Autodesk Inventor part; units mm, degrees
ref_plane "Plano de trabajo2" through (171, -60, 0) normal (1, 0, 0) x (0, 0, -1)
ref_plane "YZ Plane" through (0, 0, 0) normal (1, 0, 0) x (0, 1, 0)
ref_plane "XZ Plane" through (0, 0, 0) normal (0, 1, 0) x (-1, 0, 0)
sketch "Boceto7" plane through (0, 0, 0) normal (0, 0, 1) x (1, 0, 0)
  line L0 (0, 0) -> (342, 0)
  line L1 (171, 330.115) -> (171, 0) construction
  line L2 (131.5, 347.5309) -> (210.5, 347.5309) construction
  line L3 (210.5, 330.115) -> (131.5, 330.115)
  line L4 (0, 0) -> (131.5, 330.115)
  line L5 (342, 0) -> (210.5, 330.115)
  line L6 (0, 0) -> (0, -10) construction
  line L7 (0, -10) -> (78.602, -10) construction
  line L8 (0, -10) -> (78.602, -10)
  line L9 (0, -10) -> (0, 0)
  line L10 (78.602, -10) -> (342, -10)
  line L11 (342, -10) -> (342, 0)
  line L12 (131.5, 330.115) -> (131.5, 320.115)
  line L13 (131.5, 320.115) -> (210.5, 320.115)
  line L14 (210.5, 320.115) -> (210.5, 330.115)
  line L15 (78.602, -10) -> (78.602, 0)
  line L16 (263.398, -10) -> (263.398, 0)
  line L17 (0, -10) -> (78.602, -10)
  line L18 (78.602, -10) -> (78.602, -60)
  line L19 (78.602, -60) -> (0, -60)
  line L20 (0, -60) -> (0, -10)
  line L21 (263.398, -10) -> (263.398, -60)
  line L22 (263.398, -60) -> (342, -60)
  line L23 (342, -60) -> (342, -10)
  line L24 (78.602, 0) -> (116.5722, 189.115)
  line L25 (116.5722, 189.115) -> (225.4278, 189.115)
  line L26 (225.4278, 189.115) -> (263.398, 0)
  point P0 (263.398, 0)
  point P1 (263.398, -10)
  dimension "d68" = 79
  dimension "d69" = 39.5
  dimension "d70" = 342
  dimension "d71" = 330.115
  dimension "d72" = 10
  dimension "d73" = 78.602
  dimension "d74" = 10
  dimension "d111" = 50
  dimension "d144" = 141
extrude "Extrusión5" add sketch "Boceto7" along normal blind 35 contours L4 L12 L13 L14 L5 L0 L26 L25 L24 | L0 L15 L8 L9 | L3 L14 L13 L12 | L8 L18 L19 L20 | L0 L11 L10 L16 | L10 L23 L22 L21
extrude "Extrusión6" add sketch "Boceto7" along normal blind 191 contours L0 L15 L8 L9 | L3 L14 L13 L12 | L0 L11 L10 L16
ref_plane "Plano de trabajo2" through (171, -60, 0) normal (1, 0, 0) x (0, 0, -1)
sketch "Boceto12" plane through (171, -60, 0) normal (1, 0, 0) x (0, 0, -1)
  line L0 (-35, 380.115) -> (-191, 380.115)
  line L1 (-191, 380.115) -> (-35, 249.2155)
  line L2 (-35, 390.115) -> (-35, 60)
  line L3 (-173.0135, 380.115) -> (-35, 264.3079)
  line L4 (-173.0135, 395.115) -> (-35, 279.3079)
  line L5 (-173.0135, 410.115) -> (-35, 294.3079)
  line L6 (-173.0135, 425.115) -> (-35, 309.3079)
  line L7 (-173.0135, 440.115) -> (-35, 324.3079)
  line L8 (-173.0135, 455.115) -> (-35, 339.3079)
  line L9 (-173.0135, 470.115) -> (-35, 354.3079)
  line L10 (-173.0135, 485.115) -> (-35, 369.3079)
  line L11 (-173.0135, 500.115) -> (-35, 384.3079)
  line L12 (-173.0135, 515.115) -> (-35, 399.3079)
  line L13 (-173.0135, 530.115) -> (-35, 414.3079)
  line L14 (-35, 60) -> (-35, 390.115)
  line L15 (138.0135, 380.115) -> (138.0135, 210.115) construction
  point P0 (0, 60)
  point P1 (-10, 338.3304)
  point P2 (-23.0135, 325.115)
  point P3 (-12.1268, 325.115)
  point P4 (-30, 350.1124)
  point P5 (-30.0031, 385.115)
  point P6 (-47.8794, 380.115)
  point P7 (-65.7557, 380.115)
  point P8 (-83.632, 380.115)
  point P9 (-101.5083, 380.115)
  point P10 (-119.3846, 380.115)
  point P11 (-137.2609, 380.115)
  point P12 (-155.1372, 380.115)
  dimension "d90" = 40
  dimension "d93" = 15
  dimension "d107" = 170
  dimension "d108" = 0
extrude "Extrusión9" add sketch "Boceto12" along normal mid plane 79 contours L3 L2 L1 L0 | L0 L5 L2 L4 | L0 L7 L2 L6 | L0 L9 L2 L8 | L0 L2 L10
sketch "Boceto13" plane through (0, 0, 35) normal (0, 0, 1) x (1, 0, 0)
  circle A0 centre (81.5, 169.115) radius 12.7
  circle A1 centre (66.5, 119.115) radius 12.7
  circle A2 centre (51.5, 69.115) radius 12.7
  line L0 (116.5722, 189.115) -> (225.4278, 189.115)
  line L1 (131.5, 189.2155) -> (131.5, 320.115)
  line L2 (131.5, 320.115) -> (210.5, 320.115) construction
  line L3 (171, 320.115) -> (171, 34.3684) construction
  circle A3 centre (260.5, 169.115) radius 12.7
  circle A4 centre (275.5, 119.115) radius 12.7
  circle A5 centre (290.5, 69.115) radius 12.7
  point P0 (131.5, 193.411)
  dimension "d126" = 25.4
  dimension "d127" = 25.4
  dimension "d128" = 25.4
  dimension "d129" = 20
  dimension "d130" = 50
  dimension "d131" = 50
  dimension "d132" = 50
  dimension "d133" = 65
  dimension "d134" = 80
extrude "Extrusión10" cut sketch "Boceto13" against normal up to surface (35 mm away)
sketch "Boceto16" plane through (342, -60, 0) normal (1, 0, 0) x (0, 0, -1)
  line L0 (-191, 50) -> (-191, 60)
  line L1 (0, 0) -> (-35, 0)
  line L2 (-191, 50) -> (-35, 0)
  line L3 (-35, 0) -> (-35, 50)
  line L4 (-191, 62) -> (-35, 12)
  line L5 (-191, 74) -> (-35, 24)
  line L6 (-191, 86) -> (-35, 36)
  line L7 (-191, 98) -> (-35, 48)
  line L8 (-191, 110) -> (-35, 60)
  line L9 (-35, 50) -> (-191, 50)
  point P0 (0, 60)
  point P1 (-78.68, 50)
  point P2 (-116.12, 50)
  point P3 (-153.56, 50)
  dimension "d137" = 12
extrude "Extrusión13" add sketch "Boceto16" against normal blind 79 contours L9 L4 L3 L2 | L9 L6 L3 L5
mirror "Simetría2" about plane through (171, -60, 0) normal (1, 0, 0) of "Extrusión13"
thread "Rosca1"
thread "Rosca2"
thread "Rosca3"
thread "Rosca4"
thread "Rosca5"
thread "Rosca6"
properties part number "Soporte" material "Acero inoxidable 302 AISI"
For this review, take the finished solid that the model builds, in its own axes (mm). A direction names the side the tool comes from. Round coordinates to 2 decimals unless told otherwise and drop trailing zeros. Write each loop counter-clockwise with the first axis right and the second up, starting at its lowest first coordinate (ties: lowest second). Pieces come first, ordered by that corner, then holes. Notation, with made-up numbers: (43, 8) -> (95, 8) arc R25 ccw to (95, 43) -> close; hole circle Ø6 at (61.5, 74.5). An arc over 180 degrees is marked (long way). One line per question, with ' | ' between items. Start each with the question number.
1) Add section C-C (z = 26.5). Write out the cut boundary in (x, y) (3 decimals), and give its area (3 significant figures).
2) Wall thickness on line 1 along Y through (x, z) = (17, 48); line 2 along Y through (x, z) = (309, 59); line 3 along X through (y, z) = (-3, 13): over which ranges is each line inside the solid? List them lowest first.
3) Add section D-D (x = 241.5). Write out the cut boundary in (y, z), and give its area (3 significant figures).
4) Add section B-B (y = 32.5). Write out the cut boundary in (x, z), and give its area (3 significant figures).
5) Add section A-A (y = 161). Write out the cut boundary in (x, z), and give its area (3 significant figures).
6) Machinability: for faces 1 (the flat face through (263, -21, 67)), 2 (the flat face through (39, 0, 112)), 3 (the flat face through (78.602, -8, 53)), which of the approach directions +Z, -Z, +X, -X, +Y, -Y give a long, thin tool a straight path to every point of the face, cutting with its end or side? Answer none if there is none.
7) Mouldability with a two-part tool opening along Z and no side actions: class faces 4 (the flat face through (303.053, -22.818, 76.128)), 5 (the flat face through (38.95, -35.35, 111.91)), 6 (the flat face through (170.45, 270.42, 95.91)), 7 (the cylindrical face through (57.36, 57.85, 17.74)) as +Z half, -Z half, draft (parallel to the pull), parting line (faces both ways), or undercut.
8) For pin 1 Ø1.5 at (x, z) = (179.5, 58.5) entering from -Y (3 decimals); pin 2 Ø1.5 at (y, z) = (211.5, 34.5) entering from +X; pin 3 Ø3 at (x, y) = (157.5, 269.5) entering from +Z; pin 4 Ø20.5 at (x, y) = (66.5, 119.115) entering from +Z, all flat-tipped, find the tip position at first contact; note any pin that passes through.
Reported:
1) outline: (0, -60) -> (78.602, -60) -> (78.602, 0) -> (116.572, 189.115) -> (225.428, 189.115) -> (263.398, 0) -> (263.398, -60) -> (342, -60) -> (342, 0) -> (210.5, 330.115) -> (131.5, 330.115) -> (0, 0) -> close; hole circle Ø25.4 at (51.5, 69.115); hole circle Ø25.4 at (66.5, 119.115); hole circle Ø25.4 at (81.5, 169.115); hole circle Ø25.4 at (260.5, 169.115); hole circle Ø25.4 at (275.5, 119.115); hole circle Ø25.4 at (290.5, 69.115) | area: 48,100 mm²
2) line 1: y = -55.83 to -43.83, -31.83 to -19.83, -10 to 0 | line 2: y = -52.31 to -40.31, -28.31 to -16.31, -10 to 0 | line 3: x = 0 to 78.6, 263.4 to 342
3) outline: (109.07, 0) -> (252.29, 0) -> (252.29, 35) -> (109.07, 35) -> close | area: 5,010 mm²
4) outline: (12.95, 0) -> (85.13, 0) -> (85.13, 35) -> (12.95, 35) -> close; (256.87, 0) -> (329.05, 0) -> (329.05, 35) -> (256.87, 35) -> close | area: 5,050 mm²
5) outline: (64.13, 0) -> (71.73, 0) -> (71.73, 35) -> (64.13, 35) -> close; (91.27, 0) -> (110.93, 0) -> (110.93, 35) -> (91.27, 35) -> close; (231.07, 0) -> (250.73, 0) -> (250.73, 35) -> (231.07, 35) -> close; (270.27, 0) -> (277.87, 0) -> (277.87, 35) -> (270.27, 35) -> close | area: 1,910 mm²
6) face 1: +Z, -Z, +Y, -Y | face 2: +Z, +X, -X, +Y | face 3: -Z
7) face 4: undercut | face 5: +Z half | face 6: undercut | face 7: draft
8) pin 1: stops at y = 208.305 | pin 2: stops at x = 258.05 | pin 3: stops at z = 132.47 | pin 4: passes through
